from build123d import *

# Parameters (mm, degrees)
SKIZZE1_W                            = 77.5
SKIZZE1_H                            = 29
AUFSATZ_LINEAR_AUSTRAGEN1_DEPTH      = 15
SKIZZE2_W                            = 73.5
SKIZZE2_H                            = 9
SCHNITT_LINEAR_AUSTRAGEN2_DEPTH      = 27
SKIZZE3_W                            = 14
SKIZZE3_H                            = 3.775324495
SCHNITT_LINEAR_AUSTRAGEN3_DEPTH      = 27
SKIZZE4_R                            = 9.3
AUFSATZ_LINEAR_AUSTRAGEN2_DEPTH      = 4
SCHNITT_LINEAR_AUSTRAGEN4_DEPTH      = 4
SCHNITT_LINEAR_AUSTRAGEN4_DEPTH_BACK = 4
SKIZZE5_R                            = 6.3
GEWINDE1_PITCH                       = 1.5
SKIZZE8_R                            = 6.762792794
SCHNITT_LINEAR_AUSTRAGEN5_DEPTH      = 3
SKIZZE9_R                            = 8.045184368
SCHNITT_LINEAR_AUSTRAGEN6_DEPTH      = 3


with BuildPart() as part:
    # Skizze1 → Aufsatz-Linear austragen1 (new body)
    with BuildSketch(Plane.XY):
        Rectangle(SKIZZE1_W, SKIZZE1_H)
    extrude(amount=AUFSATZ_LINEAR_AUSTRAGEN1_DEPTH)

    # Skizze2 → Schnitt-Linear austragen2 (cut)
    with BuildSketch(Plane(origin=(0, 14.5, 0), x_dir=(1, 0, 0), z_dir=(0, 1, 0))):
        with Locations((0, -8.5)):
            Rectangle(SKIZZE2_W, SKIZZE2_H)
    extrude(amount=-SCHNITT_LINEAR_AUSTRAGEN2_DEPTH, mode=Mode.SUBTRACT)

    # Skizze3 → Schnitt-Linear austragen3 (cut)
    with BuildSketch(Plane(origin=(0, 14.5, 0), x_dir=(1, 0, 0), z_dir=(0, 1, 0))):
        with Locations((-21.75, -4.887662247)):
            Rectangle(SKIZZE3_W, SKIZZE3_H)
    extrude(amount=-SCHNITT_LINEAR_AUSTRAGEN3_DEPTH, mode=Mode.SUBTRACT)

    # Skizze4 → Aufsatz-Linear austragen2 (add)
    with BuildSketch(Plane.XY.offset(3)):
        with Locations((-21.75, 10.7)):
            Circle(SKIZZE4_R)
    extrude(amount=-AUFSATZ_LINEAR_AUSTRAGEN2_DEPTH)

    # Skizze5 → Schnitt-Linear austragen4 (cut, two sides: drawn at the far end of the back side and taken through both)
    with BuildSketch(Plane(origin=(0, 0, 0), x_dir=(-1, 0, 0), z_dir=(0, 0, -1)).offset(-SCHNITT_LINEAR_AUSTRAGEN4_DEPTH_BACK)):
        with Locations((21.75, 10.7)):
            Circle(SKIZZE5_R)
    extrude(amount=SCHNITT_LINEAR_AUSTRAGEN4_DEPTH + SCHNITT_LINEAR_AUSTRAGEN4_DEPTH_BACK, mode=Mode.SUBTRACT)

    # Gewinde1: the profile of Gewindeprofil1 profile screwed along a right-hand helix of 3.333333 turns, 8 arcs to a turn; built about Z, then put on its axis
    gewinde1_z = Axis((0, 0, 0), (0, 0, 1))
    gewinde1_corners = [(6.3003, 0, -0.000173205), (6.3003, 0, 1.312673201), (5.488101188, 0, 0.843749998), (5.488101188, 0, 0.468749998)]
    with BuildLine(mode=Mode.PRIVATE) as gewinde1_profile:
        Line(gewinde1_corners[0], gewinde1_corners[1])
        Line(gewinde1_corners[1], gewinde1_corners[2])
        Line(gewinde1_corners[2], gewinde1_corners[3])
        Line(gewinde1_corners[3], gewinde1_corners[0])
    gewinde1_cap = Face(gewinde1_profile.wire())
    gewinde1_turn_angles = [0, 22.5, 45, 67.5, 90, 112.5, 135, 157.5, 180, 202.5, 225, 247.5, 270, 292.5, 315, 337.5, 360]
    gewinde1_turn_weights = [1, 0.9238795325112867, 1, 0.9238795325112867, 1, 0.9238795325112867, 1, 0.9238795325112867, 1, 0.9238795325112867, 1, 0.9238795325112867, 1, 0.9238795325112867, 1, 0.9238795325112867, 1]
    gewinde1_turn_rails = [Edge.make_bspline([Vector(p[0], p[1], 0).rotate(gewinde1_z, gewinde1_turn_angles[k]) / gewinde1_turn_weights[k] + Vector(0, 0, p[2] + GEWINDE1_PITCH * gewinde1_turn_angles[k] / 360) for k in range(17)], [0, 0, 0, 1, 1, 2, 2, 3, 3, 4, 4, 5, 5, 6, 6, 7, 7, 8, 8, 8], 2, gewinde1_turn_weights) for p in gewinde1_corners]
    gewinde1_turn_sides = [Face.make_surface_from_curves(gewinde1_turn_rails[p[0]], gewinde1_turn_rails[p[1]]) for p in [(0, 1), (1, 2), (2, 3), (3, 0)]]
    gewinde1_last_angles = [1080, 1102.5, 1125, 1147.5, 1170, 1185, 1200]
    gewinde1_last_weights = [1, 0.9238795325112867, 1, 0.9238795325112867, 1, 0.9659258262890688, 1]
    gewinde1_last_rails = [Edge.make_bspline([Vector(p[0], p[1], 0).rotate(gewinde1_z, gewinde1_last_angles[k]) / gewinde1_last_weights[k] + Vector(0, 0, p[2] + GEWINDE1_PITCH * gewinde1_last_angles[k] / 360) for k in range(7)], [0, 0, 0, 1, 1, 2, 2, 3, 3, 3], 2, gewinde1_last_weights) for p in gewinde1_corners]
    gewinde1_last_sides = [Face.make_surface_from_curves(gewinde1_last_rails[p[0]], gewinde1_last_rails[p[1]]) for p in [(0, 1), (1, 2), (2, 3), (3, 0)]]
    gewinde1 = Plane(origin=(-21.75, 10.7, -2.6), x_dir=(1, 0, 0), z_dir=(0, 0, 1)) * Solid(Shell([*[p.moved(Location((0, 0, GEWINDE1_PITCH * i))) for i in range(3) for p in gewinde1_turn_sides], *gewinde1_last_sides, gewinde1_cap, gewinde1_cap.rotate(gewinde1_z, 1200).moved(Location((0, 0, GEWINDE1_PITCH * 1200 / 360)))]))
    add(gewinde1)

    # Skizze8 → Schnitt-Linear austragen5 (cut)
    with BuildSketch(Plane.XY.offset(3)):
        with Locations((-21.75, 10.7)):
            Circle(SKIZZE8_R)
    extrude(amount=SCHNITT_LINEAR_AUSTRAGEN5_DEPTH, mode=Mode.SUBTRACT)

    # Skizze9 → Schnitt-Linear austragen6 (cut)
    with BuildSketch(Plane(origin=(0, 0, -1), x_dir=(-1, 0, 0), z_dir=(0, 0, -1))):
        with Locations((21.75, 10.7)):
            Circle(SKIZZE9_R)
    extrude(amount=SCHNITT_LINEAR_AUSTRAGEN6_DEPTH, mode=Mode.SUBTRACT)


solid = part.part
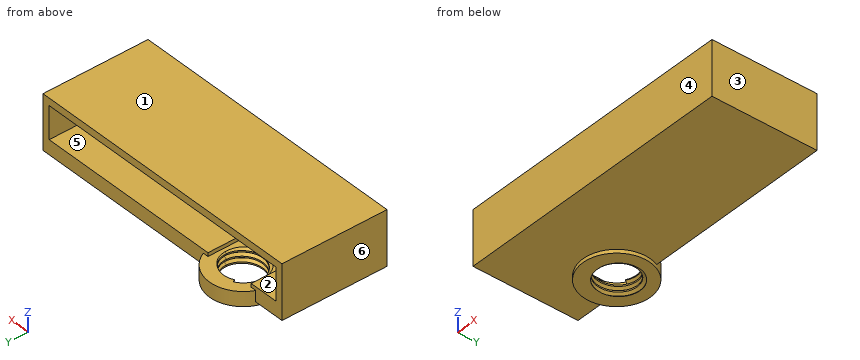
Geometry: final body of the model. Coordinates: model frame, mm. Face numbers are marked on the shaded views. A direction names the side the tool comes from. Coordinates: 2 decimals unless noted, no trailing zeros. Order: outer loops, then holes, each group sorted by start corner. A loop starts at its lowest first (then second) coordinate and runs counter-clockwise, first axis right, second up.
(1) Material intervals for probe 1 along Z at (x, y) = (16, -4.5); probe 2 along X at (y, z) = (-10, 10.5); probe 3 along Y at (x, z) = (6, 13.25), sorted ascending.
(2) Access query for the marked faces 1 and 2. Directions: +Z, -Z, +X, -X, +Y, -Y. A direction counts if a zero-diameter tool reaches every point of the face in a straight line with its end or side. Return the directions, or none.
(3) First-contact query: pin 1 (8 mm diameter, centred on x = -10, y = -7.5, fed in from -Z); pin 2 (4.5 mm diameter, centred on x = -13.5, z = 9.5, fed in from +Y). Flat tips, straight axial feed; report the tip coordinate or a pass-through.
(4) Section query B-B (x = 14.5). Return the cut outline in (y, z), plus the area to 3 significant figures.
(5) Draft query along X for the marked faces 3, 4, 5 and 6. Return one class per face: pulls with the +X half, pulls with the -X half, needs draft (parallel to the pull), parting line crosses it, or undercut.
(6) Section query A-A (y = -4.5). Return the cut outline in (x, z), plus the area to 3 significant figures.
Solution:
1. probe 1: z = 0 to 4, 13 to 15
1. probe 2: x = -38.75 to -36.75, 36.75 to 38.75
1. probe 3: y = -14.5 to 14.5
2. face 1: +Z, +X, -X, +Y, -Y
2. face 2: +Y
3. pin 1: stops at z = 0
3. pin 2: stops at y = -12.5
4. outline: (-14.5, 0) - (14.5, 0) - (14.5, 4) - (-12.5, 4) - (-12.5, 13) - (14.5, 13) - (14.5, 15) - (-14.5, 15) - close
4. area: 192 mm2
5. face 3: pulls with the +X half
5. face 4: needs draft
5. face 5: undercut
5. face 6: pulls with the -X half
6. outline: (-38.75, 0) - (38.75, 0) - (38.75, 15) - (-38.75, 15) - close; hole (-36.75, 4) - (-28.75, 4) - (-28.75, 3) - (-14.75, 3) - (-14.75, 4) - (36.75, 4) - (36.75, 13) - (-36.75, 13) - close
6. area: 487 mm2
